Design review of the part built by this model. Coordinates are the model's own, in mm. A direction names the side the tool comes from. Round coordinates to 2 decimals unless told otherwise and drop trailing zeros. Order: outer loops, then holes, each group sorted by start corner. A loop starts at its lowest first (then second) coordinate and runs counter-clockwise, first axis right, second up. Notation, with made-up numbers: (49.25, 50.25) - (88.25, 50.25) arc R17 ccw to (88.25, 81.25) - close; hole circle Ø4 at (11, 36). An arc over 180 degrees is marked (long way). Write item = value, one per line.
from build123d import *

# Parameters (mm, degrees)
CIRCLE_R         = 2
EXTRUDE002_DEPTH = 3.2
CIRCLE001_R      = 1.15
EXTRUDE003_DEPTH = 3.2
CIRCLE002_R      = 1
EXTRUDE004_DEPTH = 3.2
CIRCLE003_R      = 1.65
EXTRUDE005_DEPTH = 1
CIRCLE004_R      = 1.65
EXTRUDE006_DEPTH = 1
RECTANGLE_W      = 15.1
RECTANGLE_H      = 6
EXTRUDE007_DEPTH = 2.2
RECTANGLE002_W   = 14.5
RECTANGLE002_H   = 14.5
EXTRUDE_DEPTH    = 1.1
RECTANGLE001_W   = 15
RECTANGLE001_H   = 15
EXTRUDE001_DEPTH = 4.5
BOX_W            = 19.2
BOX_H            = 19.2
BOX_DEPTH        = 8.2


with BuildPart() as extrude002:
    # Circle → Extrude002 (new body)
    with BuildSketch(Plane.XY):
        Circle(CIRCLE_R)
    extrude(amount=-EXTRUDE002_DEPTH)


with BuildPart() as extrude003:
    # Circle001 → Extrude003 (new body)
    with BuildSketch(Plane(origin=(-5.08, 0, 0), x_dir=(1, 0, 0), z_dir=(0, 0, 1))):
        Circle(CIRCLE001_R)
    extrude(amount=-EXTRUDE003_DEPTH)


with BuildPart() as extrude004:
    # Circle002 → Extrude004 (new body)
    with BuildSketch(Plane(origin=(5.08, 0, 0), x_dir=(1, 0, 0), z_dir=(0, 0, 1))):
        Circle(CIRCLE002_R)
    extrude(amount=-EXTRUDE004_DEPTH)


with BuildPart() as extrude005:
    # Circle003 → Extrude005 (new body)
    with BuildSketch(Plane(origin=(2.54, 5.08, 0), x_dir=(1, 0, 0), z_dir=(0, 0, 1))):
        Circle(CIRCLE003_R)
    extrude(amount=-EXTRUDE005_DEPTH)


with BuildPart() as extrude006:
    # Circle004 → Extrude006 (new body)
    with BuildSketch(Plane(origin=(-3.81, 2.54, 0), x_dir=(1, 0, 0), z_dir=(0, 0, 1))):
        Circle(CIRCLE004_R)
    extrude(amount=-EXTRUDE006_DEPTH)


with BuildPart() as extrude007:
    # Rectangle → Extrude007 (new body)
    with BuildSketch(Plane(origin=(-8.03, 0.8, -1), x_dir=(1, 0, 0), z_dir=(0, 0, 1))):
        with Locations((7.55, 3)):
            Rectangle(RECTANGLE_W, RECTANGLE_H)
    extrude(amount=-EXTRUDE007_DEPTH)


with BuildPart() as extrude_body:
    # Rectangle002 → Extrude (new body)
    with BuildSketch(Plane(origin=(-7.25, -7.25, 4), x_dir=(1, 0, 0), z_dir=(0, 0, 1))):
        with Locations((7.25, 7.25)):
            Rectangle(RECTANGLE002_W, RECTANGLE002_H)
    extrude(amount=EXTRUDE_DEPTH)


with BuildPart() as fusion:
    # Rectangle001 → Extrude001 (new body)
    with BuildSketch(Plane(origin=(-7.5, -7.5, 0), x_dir=(1, 0, 0), z_dir=(0, 0, 1))):
        with Locations((7.5, 7.5)):
            Rectangle(RECTANGLE001_W, RECTANGLE001_H)
    extrude(amount=EXTRUDE001_DEPTH)

    # Fusion: union Extrude002, Extrude003, Extrude004, Extrude005, Extrude006, Extrude007, Extrude body
    add(extrude002.part)
    add(extrude003.part)
    add(extrude004.part)
    add(extrude005.part)
    add(extrude006.part)
    add(extrude007.part)
    add(extrude_body.part)


with BuildPart() as cut:
    # Box → Box (new body)
    with BuildSketch(Plane(origin=(-9.6, -9.6, -3.2), x_dir=(1, 0, 0), z_dir=(0, 0, 1))):
        with Locations((9.6, 9.6)):
            Rectangle(BOX_W, BOX_H)
    extrude(amount=BOX_DEPTH)

    # Cut: cut Fusion
    add(fusion.part, mode=Mode.SUBTRACT)


solid = cut.part
Item 1: Take a section at C-C, the plane y = 5.08. State the section outline as (x, z) points, and give its area (3 significant figures).
Data:
outline = (-9.6, -3.2) - (-8.03, -3.2) - (-8.03, -1) - (0.89, -1) - (0.89, 0) - (-7.5, 0) - (-7.5, 4.5) - (-7.25, 4.5) - (-7.25, 5) - (-9.6, 5) - close; (4.19, -1) - (7.07, -1) - (7.07, -3.2) - (9.6, -3.2) - (9.6, 5) - (7.25, 5) - (7.25, 4.5) - (7.5, 4.5) - (7.5, 0) - (4.19, 0) - close
area = 46.2 mm2
Item 2: Take a section at D-D, the plane z = -0.75. State the section outline as (x, y) points, and give its area (3 significant figures).
Data:
outline = (-9.6, -9.6) - (9.6, -9.6) - (9.6, 9.6) - (-9.6, 9.6) - close; hole circle Ø2.3 at (-5.08, 0); hole circle Ø3.3 at (-3.81, 2.54); hole circle Ø4 at (0, 0); hole circle Ø3.3 at (2.54, 5.08); hole circle Ø2 at (5.08, 0)
area = 332 mm2
Item 3: The part is to be moulded in two halves that separate along Y. For faces 4 (the face through (9.6, 0, 1)), 5 (the face through (6, 0.8, -2)), 6 (the face through (0, -9.6, 1)), say which applies: +Y half, -Y half, draft (parallel to the pull), parting line (faces both ways), or undercut.
Data:
face_4 = draft
face_5 = undercut
face_6 = -Y half
Item 4: For faces 1 (the face through (-9.6, 0, 1)), 2 (the face through (0, 7.5, 2)), 3 (the face through (7.07, 4, -2)), list the 3-axis set-ups (+Z, -Z, +X, -X, +Y, -Y) from which the entire face can be reached by the end or side of a thin tool; tool diameter is ignored.
Data:
face_1 = +Z, -Z, -X, +Y, -Y
face_2 = none
face_3 = -Z
Item 5: Take a section at A-A, the plane z = 2. State the section outline as (x, y) points, and give its area (3 significant figures).
Data:
outline = (-9.6, -9.6) - (9.6, -9.6) - (9.6, 9.6) - (-9.6, 9.6) - close; hole (-7.5, -7.5) - (7.5, -7.5) - (7.5, 7.5) - (-7.5, 7.5) - close
area = 144 mm2
Item 6: For line 1 along X through (y, z) = (5.5, 2.75); line 2 along X through (y, z) = (0, -1.9); line 3 along Y through (x, z) = (2.54, -0.3), list the stretches that pass through material, from the lowest coordinate up. Write a range as [from, to].
Data:
line_1 = [-9.6, -7.5], [7.5, 9.6]
line_2 = [-9.6, -6.23], [-3.93, -2], [2, 4.08], [6.08, 9.6]
line_3 = [-9.6, 3.43], [6.73, 9.6]
Item 7: Insertion check: P1, Ø5, axis at x = 3, y = 3.5, coming from the -Z side; P2, Ø2, axis at x = 1.5, y = 5, coming from the +Z side. Each pin has a flat end and moves straight along its axis. Give the tip position at first contact, or say it passes through.
Data:
P1 = -1
P2 = 0
Item 8: Take a section at B-B, the plane x = 5.08. State the section outline as (y, z) points.
Data:
outline = (-9.6, -3.2) - (-1, -3.2) - (-1, 0) - (-7.5, 0) - (-7.5, 4.5) - (-7.25, 4.5) - (-7.25, 5) - (-9.6, 5) - close; (1, -1) - (6.8, -1) - (6.8, -3.2) - (9.6, -3.2) - (9.6, 5) - (7.25, 5) - (7.25, 4.5) - (7.5, 4.5) - (7.5, 0) - (1, 0) - close
